```python
from build123d import *

# Parameters (mm, degrees)
SKETCH_1_W                   = 50.5
SKETCH_1_H                   = 20
EXTRUDE_1_DEPTH              = 5
SKETCH_2_R                   = 1.6
CUT_EXTRUDE_1_DEPTH          = 5
HOLE_WIZARD_M3_1_D           = 3.4
HOLE_WIZARD_M3_1_CSINK_D     = 6.72
HOLE_WIZARD_M3_1_CSINK_ANGLE = 90
SKETCH_6_R                   = 2
CUT_EXTRUDE_2_DEPTH          = 5
FILLET_1_R                   = 2


with BuildPart() as part:
    # 草图1 → 凸台-拉伸1 (new body)
    with BuildSketch(Plane.XY):
        with Locations((25.25, -10)):
            Rectangle(SKETCH_1_W, SKETCH_1_H)
    extrude(amount=EXTRUDE_1_DEPTH)

    # 草图2 → 切除-拉伸1 (cut)
    with BuildSketch(Plane(origin=(0, 0, 0), x_dir=(-1, 0, 0), z_dir=(0, 0, -1))):
        with Locations((-40.25, -5)):
            Circle(SKETCH_2_R)
        with Locations((-40.25, -15)):
            Circle(SKETCH_2_R)
        with Locations((-10.25, -5)):
            Circle(SKETCH_2_R)
        with Locations((-10.25, -15)):
            Circle(SKETCH_2_R)
    extrude(amount=-CUT_EXTRUDE_1_DEPTH, mode=Mode.SUBTRACT)

    # M3 六角凹锥坑螺钉的锥形沉头孔1 (through all)
    with Locations(Plane.XY.offset(5)):
        with Locations((10.25, -5), (10.25, -15), (40.25, -5), (40.25, -15)):
            CounterSinkHole(HOLE_WIZARD_M3_1_D / 2, HOLE_WIZARD_M3_1_CSINK_D / 2, counter_sink_angle=HOLE_WIZARD_M3_1_CSINK_ANGLE)

    # 草图6 → 切除-拉伸2 (cut)
    with BuildSketch(Plane.XY.offset(5)):
        with Locations((25.25, -3)):
            Circle(SKETCH_6_R)
        with Locations((32.25, -10)):
            Circle(SKETCH_6_R)
        with Locations((18.25, -10)):
            Circle(SKETCH_6_R)
        with Locations((25.25, -17)):
            Circle(SKETCH_6_R)
    extrude(amount=-CUT_EXTRUDE_2_DEPTH, mode=Mode.SUBTRACT)

    # 圆角1
    fillet_1_edges = [part.edges().sort_by_distance(p)[0] for p in [
        (0, 0, 2.5),
        (50.5, 0, 2.5),
        (50.5, -20, 2.5),
        (0, -20, 2.5),
    ]]
    fillet(fillet_1_edges, radius=FILLET_1_R)


solid = part.part
```
Can you work these out from the model? Positions are in its coordinate system, mm. Give positions to 0.01 mm unless a question says otherwise; leave off trailing zeros. Write each loop counter-clockwise with the first axis right and the second up, starting at its lowest first coordinate (ties: lowest second). Pieces come first, ordered by that corner, then holes. Notation, with made-up numbers: (-18.75, 50) -> (0.25, 50) arc R20 ccw to (0.25, 55) -> close; hole circle Ø11 at (23, -26). An arc over 180 degrees is marked (long way). One line per item, written item: value.
Q1. Imagine slicing it at B-B on x = 25.25. Please give me the cut outline in (y, z).
Results found:
outline: (-20, 0) -> (-19, 0) -> (-19, 5) -> (-20, 5) -> close; (-15, 0) -> (-5, 0) -> (-5, 5) -> (-15, 5) -> close; (-1, 0) -> (0, 0) -> (0, 5) -> (-1, 5) -> close
Q2. Imagine slicing it at C-C on z = 0.9. Give the number of separate pieces and of enclosed holes in the cut face, and give its area (3 significant figures).
Results found:
separate pieces: 1
enclosed holes: 8
area: 920 mm^2
Q3. Please list where these lines run through material, in increasing order: line 1 (Y direction, x = 25.25, z = 1.7); line 2 (Y direction, x = 40.25, z = 0.7); line 3 (Y direction, x = 18.25, z = 1.75). Write a range as [from, to].
Results found:
line 1: y = [-20, -19], [-15, -5], [-1, 0]
line 2: y = [-20, -16.7], [-13.3, -6.7], [-3.3, 0]
line 3: y = [-20, -12], [-8, 0]
Q4. We'd pull the mould along X, two halves only. Please class faces 1 (the face through (8.63, -14.49, 1.65)), 2 (the face through (49.9, -0.57, 2.54)), 3 (the face through (25, 0, 2)), 4 (the face through (0, -10, 2)): +X half, -X half, draft (parallel to the pull), parting line (faces both ways), or undercut.
Results found:
face 1: undercut
face 2: +X half
face 3: draft
face 4: -X half
Q5. For P1, Ø4.5, axis at x = 40.25, y = -15, coming from the +Z side, with a flat end and sliding along its axis, tell me the tip position at first contact or that it passes through.
Results found:
P1: stops at z = 3.89
Q6. Imagine slicing it at D-D on y = -10. Please give me the cut outline in (x, z).
Results found:
outline: (0, 0) -> (16.25, 0) -> (16.25, 5) -> (0, 5) -> close; (20.25, 0) -> (30.25, 0) -> (30.25, 5) -> (20.25, 5) -> close; (34.25, 0) -> (50.5, 0) -> (50.5, 5) -> (34.25, 5) -> close
Q7. Imagine slicing it at A-A on x = 32.25. Please give me the cut outline in (y, z).
Results found:
outline: (-20, 0) -> (-12, 0) -> (-12, 5) -> (-20, 5) -> close; (-8, 0) -> (0, 0) -> (0, 5) -> (-8, 5) -> close
